from build123d import *

# Parameters (mm, degrees)
BOSS_EXTRUDE1_DEPTH      = 40
SKETCH2_R                = 4
SKETCH2_R_2              = 3
CUT_EXTRUDE2_DEPTH       = 2
CUT_EXTRUDE8_DEPTH       = 114.194522836
CUT_EXTRUDE8_DEPTH_BACK  = 2
SKETCH5_R                = 3
CUT_EXTRUDE9_DEPTH       = 2
SKETCH6_R                = 3
CUT_EXTRUDE10_DEPTH      = 2
CUT_EXTRUDE11_DEPTH      = 114.194522836
CUT_EXTRUDE11_DEPTH_BACK = 2


with BuildPart() as part:
    # MetalPart → Boss-Extrude1 (new body)
    with BuildSketch(Plane.XY):
        Polygon((0, 0), (-33.5, 0), (-33.5, 82), (-31.5, 82), (-31.5, 2), (31.5, 2), (31.5, 82), (33.5, 82), (33.5, 0), align=None)
    extrude(amount=BOSS_EXTRUDE1_DEPTH)

    # Sketch2 → Cut-Extrude2 (cut)
    with BuildSketch(Plane.XZ):
        with Locations((0, 20)):
            Circle(SKETCH2_R)
        with Locations((-13, 28)):
            Circle(SKETCH2_R_2)
        with Locations((13, 12)):
            Circle(SKETCH2_R_2)
    extrude(amount=-CUT_EXTRUDE2_DEPTH, mode=Mode.SUBTRACT)

    # Sketch3 → Cut-Extrude8 (cut, two sides: drawn at the far end of the back side and taken through both)
    with BuildSketch(Plane(origin=(33.5, 0, 0), x_dir=(0, 0, -1), z_dir=(1, 0, 0)).offset(-CUT_EXTRUDE8_DEPTH_BACK)):
        with BuildLine():
            Line((-206.064089399, 67), (-40, 67))
            Line((-40, 67), (-35, 67))
            ThreePointArc((-35, 67), (-20, 82), (-5, 67))
            Line((-5, 67), (0, 67))
            Line((0, 67), (166.064089399, 67))
            Line((166.064089399, 67), (166.064089399, 399.128178798))
            Line((166.064089399, 399.128178798), (-206.064089399, 399.128178798))
            Line((-206.064089399, 399.128178798), (-206.064089399, 67))
        make_face()
    extrude(amount=CUT_EXTRUDE8_DEPTH + CUT_EXTRUDE8_DEPTH_BACK, mode=Mode.SUBTRACT)

    # Sketch5 → Cut-Extrude9 (cut)
    with BuildSketch(Plane(origin=(33.5, 0, 0), x_dir=(0, 0, -1), z_dir=(1, 0, 0))):
        with Locations((-9, 55)):
            Circle(SKETCH5_R)
        with Locations((-31, 32.5)):
            Circle(SKETCH5_R)
    extrude(amount=-CUT_EXTRUDE9_DEPTH, mode=Mode.SUBTRACT)

    # Sketch6 → Cut-Extrude10 (cut)
    with BuildSketch(Plane.ZY.offset(33.5)):
        with Locations((9, 32.5)):
            Circle(SKETCH6_R)
        with Locations((31, 55)):
            Circle(SKETCH6_R)
    extrude(amount=-CUT_EXTRUDE10_DEPTH, mode=Mode.SUBTRACT)

    # Sketch7 → Cut-Extrude11 (cut, two sides: drawn at the far end of the back side and taken through both)
    with BuildSketch(Plane.ZY.offset(33.5).offset(-CUT_EXTRUDE11_DEPTH_BACK)):
        with BuildLine():
            Line((-166.064089399, 67), (0, 67))
            Line((0, 67), (5, 67))
            ThreePointArc((5, 67), (20, 82), (35, 67))
            Line((35, 67), (40, 67))
            Line((40, 67), (206.064089399, 67))
            Line((206.064089399, 67), (206.064089399, 399.128178798))
            Line((206.064089399, 399.128178798), (-166.064089399, 399.128178798))
            Line((-166.064089399, 399.128178798), (-166.064089399, 67))
        make_face()
    extrude(amount=CUT_EXTRUDE11_DEPTH + CUT_EXTRUDE11_DEPTH_BACK, mode=Mode.SUBTRACT)


solid = part.part
Read the model definition and answer for the solid it produces. Units are mm, in the model's axes. A direction names the side the tool comes from. Give positions to 0.01 mm unless a question says otherwise; leave off trailing zeros. Loops run counter-clockwise (first coordinate to the right, second up) from the corner with the lowest first, then second, coordinate; pieces in that order, holes last. Notation, with made-up numbers: M 33,-35.75 L 85,-35.75 A26 ccw 85,-16.75 Z; hole C 4,-33 d2. An arc over 180 degrees is marked long. Write each question's results on one line, items separated by ' | '.
1. Straight lines are drawn through the part: line 1 (Z direction, x = -13, y = 1.5); line 2 (Z direction, x = 0, y = 1.65); line 3 (X direction, y = 11.5, z = 20). For each, find the intervals that lie inside material, in ascending order. Write a range as [from, to].
Values:
line 1: z = [0, 25], [31, 40] | line 2: z = [0, 16], [24, 40] | line 3: x = [-33.5, -31.5], [31.5, 33.5]
2. The mould has two halves that part along Z. Classify faces 4 (the face through (32, 82, 20)), 5 (the face through (33.5, 42, 20)), 6 (the face through (10.6, 1, 10.2)): pulls with the +Z half, pulls with the -Z half, needs draft (parallel to the pull), parting line crosses it, or undercut.
Values:
face 4: parting line crosses it | face 5: needs draft | face 6: undercut
3. Section C-C on y = 25 is taken. Give the vertices of the cut face in (x, z).
Values:
outline: M -33.5,0 L -31.5,0 L -31.5,40 L -33.5,40 Z; M 31.5,0 L 33.5,0 L 33.5,40 L 31.5,40 Z
4. A tool of negligible diameter and unlimited length cuts with its end or side. For faces 1 (the face through (-31.5, 43, 20)), 2 (the face through (-32.51, 35.03, 10.61)), 3 (the face through (-32, 67, 37)), from which of +Z, -Z, +X, -X, +Y, -Y can it reach the whole face along a straight path? Write none if from no direction.
Values:
face 1: +Z, -Z, +Y | face 2: -X | face 3: +Z, +X, -X, +Y
5. Section A-A on z = 20 is taken. Give the vertices of the cut face in (x, y), plus the area to 3 significant figures.
Values:
outline: M -33.5,0 L -4,0 L -4,2 L -31.5,2 L -31.5,82 L -33.5,82 Z; M 4,0 L 33.5,0 L 33.5,82 L 31.5,82 L 31.5,2 L 4,2 Z | area: 438 mm^2
6. Given pin 1 (1 mm diameter, centred on x = -32, z = 37, fed in from +Y); pin 2 (6 mm diameter, centred on x = -1.5, z = 15.5, fed in from +Y), each flat-ended and moving along its own axis, determine where each tip first touches the part or whether it passes through.
Values:
pin 1: stops at y = 67 | pin 2: stops at y = 2
7. Section B-B on x = 13 is taken. Give the vertices of the cut face in (y, z).
Values:
outline: M 0,0 L 2,0 L 2,9 L 0,9 Z; M 0,15 L 2,15 L 2,40 L 0,40 Z
8. Section D-D on y = 34 is taken. Give the vertices of the cut face in (x, z).
Values:
outline: M -33.5,0 L -31.5,0 L -31.5,6.4 L -33.5,6.4 Z; M -33.5,11.6 L -31.5,11.6 L -31.5,40 L -33.5,40 Z; M 31.5,0 L 33.5,0 L 33.5,28.4 L 31.5,28.4 Z; M 31.5,33.6 L 33.5,33.6 L 33.5,40 L 31.5,40 Z
